Can you work these out from the model? Positions are in its coordinate system, mm. Face numbers are marked on the shaded views. A direction names the side the tool comes from. Give positions to 0.01 mm unless a question says otherwise; leave off trailing zeros. Order: outer loops, then holes, each group sorted by start corner. A loop starts at its lowest first (then second) coordinate and runs counter-clockwise, first axis right, second up. Notation, with made-up numbers: (21, -12) -> (55, -12) arc R34 cw to (55, 18) -> close; hole circle Ø11 at (28, 42). An arc over 180 degrees is marked (long way). Answer as CSV lines item,"result".
```python
from build123d import *

# Parameters (mm, degrees)
BOSS_EXTRUDE1_DEPTH    = 2
SKETCHED_START         = -17.446464646
SKETCHED_BEND2_DEPTH   = 25.4
SKETCHED_BEND2_2_DEPTH = 25.4


# Read off the part's stored shape, not the designer's step: Sketched Bend2
with BuildPart() as part:
    # Sketch1 → Boss-Extrude1 (new body)
    with BuildSketch(Plane.XY):
        Polygon((-17.446464646, 32.712121212), (7.953535354, 32.712121212), (7.953535354, 7.825252525), (7.953535354, -18.087878788), (-17.446464646, -18.087878788), align=None)
    extrude(amount=BOSS_EXTRUDE1_DEPTH)

    # Sketched Bend2 outline → Sketched Bend2 (cut)
    with BuildSketch(Plane.YZ.offset(SKETCHED_START)):
        with BuildLine():
            ThreePointArc((11.852121212, 0), (9.721393637, 0.531059991), (8.089143668, 2))
            Line((8.089143668, 2), (-18.087878788, 2))
            Line((-18.087878788, 2), (-18.087878788, 0))
            Line((-18.087878788, 0), (11.852121212, 0))
        make_face()
    extrude(amount=SKETCHED_BEND2_DEPTH, mode=Mode.SUBTRACT)

    # Sketched Bend2 2 outline → Sketched Bend2 2 (add)
    with BuildSketch(Plane.YZ.offset(SKETCHED_START)):
        with BuildLine():
            Line((9.312121212, 4.54), (9.312121212, 28.919381003))
            Line((9.312121212, 28.919381003), (7.312121212, 28.919381003))
            Line((7.312121212, 28.919381003), (7.312121212, 4.54))
            ThreePointArc((7.312121212, 4.54), (7.510720629, 3.211903251), (8.089143668, 2))
            Line((8.089143668, 2), (11.852121212, 2))
            ThreePointArc((11.852121212, 2), (10.056069988, 2.743948776), (9.312121212, 4.54))
        make_face()
    extrude(amount=SKETCHED_BEND2_2_DEPTH)


solid = part.part
```
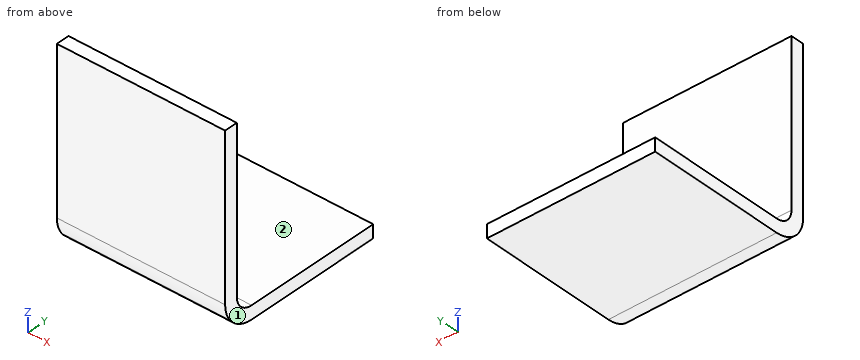
Item 1: For pin 1 (7.5 mm diameter, centred on x = -10, z = 15.5, fed in from +Y); pin 2 (6.5 mm diameter, centred on x = -10, y = 17.5, fed in from +Z), each with a flat end and sliding along its axis, tell me the tip position at first contact or that it passes through.
Numbers:
pin 1,"stops at y = 9.31"
pin 2,"stops at z = 2"
Item 2: Imagine slicing it at A-A, the plane x = -1. Please give me the cut outline in (y, z), then the cut area to 3 significant figures.
Numbers:
outline,"(7.31, 4.54) arc R4.54 ccw to (11.85, 0) -> (32.71, 0) -> (32.71, 2) -> (11.85, 2) arc R2.54 cw to (9.31, 4.54) -> (9.31, 28.92) -> (7.31, 28.92) -> close"
area,"102 mm²"
Item 3: Please list where these lines run through material, in increasing order: line 1 along Y through (x, z) = (2.5, 11.5); line 2 along Z through (x, y) = (0.5, 28.5); line 3 along Z through (x, y) = (-10, 9).
Numbers:
line 1,"y = 7.31 to 9.31"
line 2,"z = 0 to 2"
line 3,"z = 1.01 to 28.92"
Item 4: Imagine slicing it at C-C, the plane y = 14.25. Please give me the cut outline in (x, z), then the cut area to 3 significant figures.
Numbers:
outline,"(-17.45, 0) -> (7.95, 0) -> (7.95, 2) -> (-17.45, 2) -> close"
area,"50.8 mm²"
Item 5: Imagine slicing it at B-B, the plane z = 19. Please give me the cut outline in (x, y).
Numbers:
outline,"(-17.45, 7.31) -> (7.95, 7.31) -> (7.95, 9.31) -> (-17.45, 9.31) -> close"
Item 6: For the marked faces 1 and 2, which set-ups out of +Z, -Z, +X, -X, +Y, -Y let a thin tool reach every point of the face, with its end or its side?
Numbers:
face 1,"+Z, -Z, +X, +Y, -Y"
face 2,"+Z, +X, -X, +Y"
